```python
from build123d import *

# Parameters (mm, degrees)
SKETCH1_W           = 200
SKETCH1_H           = 200
BOSS_EXTRUDE1_DEPTH = 10


with BuildPart() as part:
    # Sketch1 → Boss-Extrude1 (new body)
    with BuildSketch(Plane(origin=(0, 0, 0), x_dir=(1, 0, 0), z_dir=(0, 1, 0))):
        with Locations((230, -230)):
            Rectangle(SKETCH1_W, SKETCH1_H)
        with BuildLine():
            Line((130, -330), (130, -277.5))
            Line((130, -277.5), (0, -407.5))
            ThreePointArc((0, -407.5), (0, -460), (52.5, -460))
            Line((52.5, -460), (182.5, -330))
            Line((182.5, -330), (130, -330))
        make_face()
        with BuildLine():
            Line((130, -130), (182.5, -130))
            Line((182.5, -130), (52.5, 0))
            ThreePointArc((52.5, 0), (0, 0), (0, -52.5))
            Line((0, -52.5), (130, -182.5))
            Line((130, -182.5), (130, -130))
        make_face()
        with BuildLine():
            Line((407.5, 0), (277.5, -130))
            Line((277.5, -130), (330, -130))
            Line((330, -130), (330, -182.5))
            Line((330, -182.5), (460, -52.5))
            ThreePointArc((460, -52.5), (460, 0), (407.5, 0))
        make_face()
        with BuildLine():
            Line((460, -407.5), (330, -277.5))
            Line((330, -277.5), (330, -330))
            Line((330, -330), (277.5, -330))
            Line((277.5, -330), (407.5, -460))
            ThreePointArc((407.5, -460), (460, -460), (460, -407.5))
        make_face()
    extrude(amount=BOSS_EXTRUDE1_DEPTH)


solid = part.part
```
Part model, mm, in its own coordinate system. A direction names the side the tool comes from. Round coordinates to 2 decimals unless told otherwise and drop trailing zeros. Loops run counter-clockwise (first coordinate to the right, second up) from the corner with the lowest first, then second, coordinate; pieces in that order, holes last.
1. Drill centre lines: line 1 along X through (y, z) = (2.75, 251); line 2 along X through (y, z) = (9.25, 71.5). Where is each one in solid material? Low to high.
Solutions:
line 1: x = 130 to 330
line 2: x = 19 to 124, 336 to 441
2. Slice it at C-C (y = 7). Give the cut face in (x, z), and give its area (3 significant figures).
Solutions:
outline: (0, 52.5) arc R37.12 ccw to (52.5, 0) - (182.5, 130) - (277.5, 130) - (407.5, 0) arc R37.12 ccw to (460, 52.5) - (330, 182.5) - (330, 277.5) - (460, 407.5) arc R37.12 ccw to (407.5, 460) - (277.5, 330) - (182.5, 330) - (52.5, 460) arc R37.12 ccw to (0, 407.5) - (130, 277.5) - (130, 182.5) - close
area: 97,700 mm2
3. Slice it at A-A (z = 388). Give the cut face in (x, y), and give its area (3 significant figures).
Solutions:
outline: (19.5, 0) - (124.5, 0) - (124.5, 10) - (19.5, 10) - close; (335.5, 0) - (440.5, 0) - (440.5, 10) - (335.5, 10) - close
area: 2,100 mm2
4. Slice it at D-D (z = 251). Give the cut face in (x, y), and give its area (3 significant figures).
Solutions:
outline: (130, 0) - (330, 0) - (330, 10) - (130, 10) - close
area: 2,000 mm2
5. 3-axis set-ups, long thin cutter, end or side, ignore diameter. For faces 5 (the face through (118.4, 4.9, 65.9)), 6 (the face through (64.1, 4.9, 116.6)), 7 (the face through (395.9, 4.9, 343.4)): which of +Z, -Z, +X, -X, +Y, -Y reach the whole face in a straight line?
Solutions:
face 5: -Z, +Y, -Y
face 6: -X, +Y, -Y
face 7: +X, +Y, -Y
6. Flat gauge pins, fed straight in: pin 1 (1 mm diameter, centred on x = 412.5, y = 1, fed in from -Z); pin 2 (3 mm diameter, centred on x = 247.5, y = 5, fed in from +Z); pin 3 (5 mm diameter, centred on x = 38, y = 6.5, fed in from +Z). Where does each tip first touch, or does it go through?
Solutions:
pin 1: stops at z = -4.53
pin 2: stops at z = 330
pin 3: stops at z = 469.7
7. Two-plate mould, pull along X, no slides. Class faces 1 (the face through (459.42, 4.93, 460.57)), 2 (the face through (341.6, 4.9, 394.1)), 3 (the face through (65.9, 4.9, 341.6)), 4 (the face through (247, 0, 229)): pulls with the +X half, pulls with the -X half, needs draft (parallel to the pull), parting line crosses it, or undercut.
Solutions:
face 1: undercut
face 2: undercut
face 3: pulls with the -X half
face 4: needs draft
8. Slice it at B-B (x = 345.5). Give the cut face in (y, z).
Solutions:
outline: (0, 62) - (10, 62) - (10, 167) - (0, 167) - close; (0, 293) - (10, 293) - (10, 398) - (0, 398) - close
